The model under review builds one solid part; all positions refer to its coordinate system, in mm. A direction names the side the tool comes from. Coordinates: 2 decimals unless noted, no trailing zeros. Loops run counter-clockwise (first coordinate to the right, second up) from the corner with the lowest first, then second, coordinate; pieces in that order, holes last. Notation, with made-up numbers: M -39.75,-24 L 5.25,-24 A5 cw 5.25,-19 Z; hole C -10,78 d10. An arc over 180 degrees is marked long. Write item = value, one per line. Start each with the question number.
Q1. Wall thickness on probe 1 along Y at (x, z) = (17, -25); probe 2 along Y at (x, z) = (8.5, -25); probe 3 along X at (y, z) = (-49, -25.65): over which ranges is each line inside the solid? List them lowest first.
Q2. We need section A-A on y = -49. Give the boundary of the cut face in (x, z).
Q3. Clearance check with flat-ended pins moving along their axes: pin 1 Ø4.5 at (x, y) = (17, -49) entering from +Z; pin 2 Ø10 at (x, y) = (15.5, -48.5) entering from +Z; pin 3 Ø12 at (y, z) = (-48.5, -11.5) entering from +X; pin 4 Ø11.5 at (x, y) = (16.5, -44.5) entering from +Z. State where each tip first meets the part, or that it passes through.
Q4. For faces 4 (the face through (21, -42, -11)), 5 (the face through (16, -41.75, -11)), 6 (the face through (22, -31, -25)), 7 (the face through (16, -42.75, -11)), 8 (the face through (11, -54, -25)), list the 3-axis set-ups (+Z, -Z, +X, -X, +Y, -Y) from which the entire face can be reached by the end or side of a thin tool; tool diameter is ignored.
Q5. We need section C-C on y = -44.5. Give the boundary of the cut face in (x, z).
Q6. We need section D-D on z = -19. Give the boundary of the cut face in (x, y).
Q7. We need section B-B on x = 17. Give the boundary of the cut face in (y, z), and give its area (3 significant figures).
Q8. Mouldability with a two-part tool opening along X and no side actions: class faces 1 (the face through (18, -31, -25.5)), 2 (the face through (23, -38, -25)), 3 (the face through (11, -55, -25)) as released by +X, released by -X, zero draft, split by the parting line, or undercut.
from build123d import *

# Parameters (mm, degrees)
SKETCH006_R      = 1.7
EXTRUDE004_DEPTH = 1
EXTRUDE005_DEPTH = 2
SKETCH017_R      = 3.7
SKETCH017_R_2    = 1.7
EXTRUDE014_DEPTH = 1
EXTRUDE003_DEPTH = 27.5


with BuildPart() as extrude004:
    # Sketch006 → Extrude004 (new body)
    with BuildSketch(Plane.XY.offset(10)):
        Polygon((-11, 0), (0, 0), (0, 12), (-23, 12), (-23, -21.5), (-11, -21.5), align=None)
        with Locations((-17, 6)):
            Circle(SKETCH006_R, mode=Mode.SUBTRACT)
    extrude(amount=EXTRUDE004_DEPTH)


with BuildPart() as extrude004_1:
    # Extrude004 placement: moved
    add(extrude004.part.moved(Location((0, 0, -36.5))))


with BuildPart() as extrude005:
    # Sketch007 → Extrude005 (new body)
    with BuildSketch(Plane.XY.offset(10)):
        Polygon((0, 12), (-23, 12), (-23, -21.5), (-22, -21.5), (-22, -2.25), (-13, -2.25), (-13, -21.5), (-11, -21.5), (-11, 0), (0, 0), (0, 1), (-22, 1), (-22, 11), (0, 11), align=None)
    extrude(amount=EXTRUDE005_DEPTH)


with BuildPart() as extrude005_1:
    # Extrude005 placement: moved
    add(extrude005.part.moved(Location((0, 0, -35.5))))


with BuildPart() as extrude014:
    # Sketch017 → Extrude014 (new body)
    with BuildSketch(Plane.XY.offset(10)):
        with Locations((-17, 6)):
            Circle(SKETCH017_R)
        with Locations((-17, 6)):
            Circle(SKETCH017_R_2, mode=Mode.SUBTRACT)
    extrude(amount=EXTRUDE014_DEPTH)


with BuildPart() as extrude014_1:
    # Extrude014 placement: moved
    add(extrude014.part.moved(Location((0, 0, -35.5))))


with BuildPart() as body004:
    # Sketch003 → Extrude003 (new body)
    with BuildSketch(Plane.XY):
        Polygon((-21, -0.25), (-11, -0.25), (-11, -21.5), (-12, -21.5), (-12, -1.25), (-21, -1.25), align=None)
    extrude(amount=-EXTRUDE003_DEPTH)


with BuildPart() as body004_1:
    # Extrude003 placement: moved
    add(body004.part.moved(Location((0, 0, 2))))

    # Fusion013: union Extrude004, Extrude005, Extrude014
    add(extrude004_1.part)
    add(extrude005_1.part)
    add(extrude014_1.part)


with BuildPart() as body005:
    # Part__Mirroring005: instance of Body004
    add(body004_1.part.mirror(Plane(origin=(0, 0, 0), x_dir=(0, -1, 0), z_dir=(1, 0, 0))))


with BuildPart() as part_mirroring006:
    # Part__Mirroring006: instance of Body005
    add(body005.part.mirror(Plane(origin=(0, -21.5, 0), x_dir=(1, 0, 0), z_dir=(0, 1, 0))))


solid = part_mirroring006.part
Returned:
q1.probe_1 = -55 to -54, -52.7 to -50.7, -47.3 to -45.3, -44 to -40.75
q1.probe_2 = -55 to -54, -44 to -43
q1.probe_3 = 0 to 15.3, 18.7 to 23
q2.outline = M 0,-26.5 L 15.3,-26.5 L 15.3,-24.5 L 13.3,-24.5 L 13.3,-25.5 L 0,-25.5 Z; M 18.7,-26.5 L 23,-26.5 L 23,-23.5 L 22,-23.5 L 22,-25.5 L 20.7,-25.5 L 20.7,-24.5 L 18.7,-24.5 Z
q3.pin_1 = -24.5
q3.pin_2 = -23.5
q3.pin_3 = 21
q3.pin_4 = 2
q4.face_4 = +Z, +X, +Y, -Y
q4.face_5 = +Z, +X, +Y
q4.face_6 = +Z, +Y
q4.face_7 = +Z, +X, -X, -Y
q4.face_8 = +Z, -X
q5.outline = M 0,-26.5 L 23,-26.5 L 23,-23.5 L 22,-23.5 L 22,-25.5 L 0,-25.5 Z
q6.outline = M 11,-42.75 L 21,-42.75 L 21,-41.75 L 12,-41.75 L 12,-21.5 L 11,-21.5 Z
q7.outline = M -55,-26.5 L -50.7,-26.5 L -50.7,-24.5 L -52.7,-24.5 L -52.7,-25.5 L -54,-25.5 L -54,-23.5 L -55,-23.5 Z; M -47.3,-26.5 L -21.5,-26.5 L -21.5,-25.5 L -40.75,-25.5 L -40.75,-23.5 L -41.75,-23.5 L -41.75,2 L -42.75,2 L -42.75,-23.5 L -44,-23.5 L -44,-25.5 L -45.3,-25.5 L -45.3,-24.5 L -47.3,-24.5 Z
q7.area = 68.1 mm^2
q8.face_1 = undercut
q8.face_2 = released by +X
q8.face_3 = zero draft
